from build123d import *

# Parameters (mm, degrees)
F1_DEPTH = 1000
F3_D     = 8
F4_R     = 2


# Not quite as in the source:
# - a feature names something its author has since deleted; it is built from what else it names


with BuildPart() as f1:
    # F0 (on Right) → F1 (new body)
    with BuildSketch(Plane.YZ):
        Polygon((-18.8378913403, 427.8021101952), (-18.8378913403, 404.8021101952), (-16.8378913403, 404.8021101952), (-16.8378913403, 429.8021101952), (-56.8378913403, 429.8021101952), (-56.8378913403, 79.8021101952), (-29.8378913403, 79.8021101952), (-29.8378913403, 53.8021101952), (-27.8378913403, 53.8021101952), (-27.8378913403, 81.8021101952), (-54.8378913403, 81.8021101952), (-54.8378913403, 427.8021101952), align=None)
    extrude(amount=F1_DEPTH)

    # F3 (through all)
    with Locations(Plane.XZ.offset(29.8378913403)):
        with Locations((350, 66.8021101952), (650, 66.8021101952), (900, 66.8021101952), (100, 66.8021101952)):
            Hole(F3_D / 2)

    # F4
    f4_edges = [f1.edges().sort_by_distance(p)[0] for p in [
        (500, -56.837891, 429.80211),
        (500, -16.837891, 429.80211),
        (500, -56.837891, 79.80211),
        (500, -27.837891, 81.80211),
        (500, -54.837891, 81.80211),
        (500, -29.837891, 79.80211),
        (500, -18.837891, 427.80211),
        (500, -54.837891, 427.80211),
    ]]
    fillet(f4_edges, radius=F4_R)


solid = f1.part
Model file for the job. Use its own axes, mm. A direction names the side the tool comes from. Coordinates: 2 decimals unless noted, no trailing zeros. Loops run counter-clockwise (first coordinate to the right, second up) from the corner with the lowest first, then second, coordinate; pieces in that order, holes last. Notation, with made-up numbers: (86, 61) -> (141, 61) arc R25 cw to (141, 95) -> close; hole circle Ø4 at (47, 33). An arc over 180 degrees is marked (long way). Use one line per item in the form item = value. Start each with the question number.
(1) Cut at B-B on x = 720. Give the cut face in (y, z), and give its area (3 significant figures).
(2) Pull direction Z, two halves, no side cores. Call faces 4 (the flat face through (493, -37, 427.802)), 5 (the flat face through (493, -43, 79.802)), 6 (the flat face through (493, -18.838, 415)): pulls with the +Z half, pulls with the -Z half, needs draft (parallel to the pull), parting line crosses it, or undercut.
(3) Tool access for faces 1 (the flat face through (493, -29.838, 66)), 2 (the flat face through (493, -41, 81.802)), 3 (the flat face through (493, -27.838, 67)): list every direction of +Z, -Z, +X, -X, +Y, -Y with a clear straight run to the whole face (end or side of a thin tool).
(4) Probe probe 1 along Z at (x, y) = (350, -29); probe 2 along Z at (x, y) = (100, -28.35); probe 3 along Z at (x, y) = (843, -37). List the from-to ranges inside material, lowest first. Write a range as from..to.
(5) Cut at A-A on y = -40.5. Give the cut face in (x, z).
(6) Flat gauge pins, fed straight in: pin 1 (7 mm diameter, centred on x = 650, z = 66.8, fed in from -Y); pin 2 (13 mm diameter, centred on x = 350, z = 66.8, fed in from -Y); pin 3 (9.5 mm diameter, centred on x = 522, y = -39.5, fed in from -Z); pin 4 (8 mm diameter, centred on x = 376.5, z = 379, fed in from +Y). Where does each tip first touch, or does it go through?
(7) Cut at C-C on z = 382. Give the cut face in (x, y).
Values:
q1.outline = (-56.84, 81.8) arc R2 ccw to (-54.84, 79.8) -> (-31.84, 79.8) arc R2 cw to (-29.84, 77.8) -> (-29.84, 53.8) -> (-27.84, 53.8) -> (-27.84, 79.8) arc R2 ccw to (-29.84, 81.8) -> (-52.84, 81.8) arc R2 cw to (-54.84, 83.8) -> (-54.84, 425.8) arc R2 cw to (-52.84, 427.8) -> (-20.84, 427.8) arc R2 cw to (-18.84, 425.8) -> (-18.84, 404.8) -> (-16.84, 404.8) -> (-16.84, 427.8) arc R2 ccw to (-18.84, 429.8) -> (-54.84, 429.8) arc R2 ccw to (-56.84, 427.8) -> close
q1.area = 928 mm2
q2.face_4 = undercut
q2.face_5 = pulls with the -Z half
q2.face_6 = needs draft
q3.face_1 = -Z, +X, -X, -Y
q3.face_2 = +X, -X, +Y
q3.face_3 = -Z, +X, -X, +Y
q4.probe_1 = 53.8..62.8, 70.8..81.62, 427.8..429.8
q4.probe_2 = 53.8..62.8, 70.8..81.14, 427.8..429.8
q4.probe_3 = 79.8..81.8, 427.8..429.8
q5.outline = (0, 79.8) -> (1000, 79.8) -> (1000, 81.8) -> (0, 81.8) -> close; (0, 427.8) -> (1000, 427.8) -> (1000, 429.8) -> (0, 429.8) -> close
q6.pin_1 = through
q6.pin_2 = -29.84
q6.pin_3 = 79.8
q6.pin_4 = -54.84
q7.outline = (0, -56.84) -> (1000, -56.84) -> (1000, -54.84) -> (0, -54.84) -> close
